Work out the finished part from the listing and answer in its coordinate system (mm). A direction names the side the tool comes from. Round coordinates to 2 decimals unless told otherwise and drop trailing zeros. Loops run counter-clockwise (first coordinate to the right, second up) from the corner with the lowest first, then second, coordinate; pieces in that order, holes last. Notation, with made-up numbers: (51.25, -15) -> (62.25, -15) arc R14 ccw to (62.25, -7) -> close; hole circle Ø8 at (36.5, -12.75). An arc over 180 degrees is marked (long way). Use one line per item in the form item = value.
```python
from build123d import *

# Parameters (mm, degrees)
F0_W     = 14.6
F0_H     = 15
F1_DEPTH = 15
F2_R     = 2
F3_R     = 3
F4_DEPTH = 15.001
F5_SIZE2 = 0.5
F5_SIZE  = 0.5
F9_SIZE2 = 0.5
F9_SIZE  = 0.5


# Not quite as in the source:
# - a pattern or mirror of a feature is missing from the dataset's text; its kind, count and spacing are read off the source's solid


with BuildPart() as f1:
    # F0 (on Right) → F1 (new body)
    with BuildSketch(Plane.YZ):
        Rectangle(F0_W, F0_H)
    extrude(amount=-F1_DEPTH)

    # F2
    f2_edges = [f1.edges().sort_by_distance(p)[0] for p in [
        (-7.5, -7.3, 7.5),
        (-7.5, 7.3, 7.5),
        (-7.5, -7.3, -7.5),
        (-7.5, 7.3, -7.5),
    ]]
    fillet(f2_edges, radius=F2_R)

    # F3 (on face) → F4 (cut, through all)
    with BuildSketch(Plane.YZ):
        Circle(F3_R)
    extrude(amount=-F4_DEPTH, mode=Mode.SUBTRACT)

    # F5
    f5_edges = [f1.edges().sort_by_distance(p)[0] for p in [
        (0, -3, 0),
        (-7.5, 3, 0),
        (-15, -3, 0),
    ]]
    chamfer(f5_edges, length=F5_SIZE, length2=F5_SIZE2)

    # F7 (on mid) → F8 (revolve)
    with BuildSketch(Plane.YZ.offset(-7.5)):
        Polygon((-7.3, 0), (-12.8, 0), (-12.8, -4), (-10.8, -4), (-10.8, -3), (-9.8, -3), (-9.8, -4), (-7.3, -4), align=None)
    f8 = revolve(axis=Axis((-7.5, -3.65, 0), (0, -1, 0)))

    # F8_copies: F8 across plane
    add(f8.mirror(Plane.ZX))

    # F9
    f9_edges = [f1.edges().sort_by_distance(p)[0] for p in [
        (-7.5, -12.8, 4),
        (-7.5, 12.8, 4),
    ]]
    chamfer(f9_edges, length=F9_SIZE, length2=F9_SIZE2)


solid = f1.part
```
(1) Find section C-C, the plane y = -9. Write down the section's boundary in (x, z), then the cut area to 3 significant figures.
Completed:
outline = circle Ø8 at (-7.5, 0)
area = 50.3 mm2
(2) Consider L1, parallel to Z at x = -7.75, y = 0; L2, parallel to Y at x = -9.5, z = 1; L3, parallel to Y at x = -3.75, z = -1.25. Determine where each line is inside the solid, lowest interval first.
Completed:
L1 = -7.5 to -3, 3 to 7.5
L2 = -12.8 to -2.83, 2.83 to 12.8
L3 = -12.35 to -10.8, -9.8 to -2.73, 2.73 to 9.8, 10.8 to 12.35
(3) Find section A-A, the plane y = 0. Write down the section's boundary in (x, z).
Completed:
outline = (-15, -7.5) -> (0, -7.5) -> (0, -3.5) -> (-0.5, -3) -> (-14.5, -3) -> (-15, -3.5) -> close; (-15, 3.5) -> (-14.5, 3) -> (-0.5, 3) -> (0, 3.5) -> (0, 7.5) -> (-15, 7.5) -> close
(4) Given P1, Ø3.5, axis at x = -4, z = -2, coming from the +Y side; P2, Ø1, axis at x = -12, z = 1.5, coming from the +Y side; P3, Ø5.5, axis at y = 0, z = 0, coming from the +X side, each flat-ended and moving along its own axis, determine where each tip first touches the part or whether it passes through.
Completed:
P1 = 12.8
P2 = 7.3
P3 = through
(5) Find section B-B, the plane x = -2.75. Write down the section's boundary in (y, z), then the cut area to 3 significant figures.
Completed:
outline = (-7.3, -5.5) arc R2 ccw to (-5.3, -7.5) -> (5.3, -7.5) arc R2 ccw to (7.3, -5.5) -> (7.3, 5.5) arc R2 ccw to (5.3, 7.5) -> (-5.3, 7.5) arc R2 ccw to (-7.3, 5.5) -> close; hole circle Ø6 at (0, 0)
area = 187 mm2
(6) For a pull along Y with two mould halves and no side action, classify faces 1 (the cylindrical face through (-4.526, -10.293, 0.391)), 2 (the flat face through (0, -3.3, 1.8)), 3 (the cylindrical face through (-7.6, -6.73, 6.9)) as +Y half, -Y half, draft (parallel to the pull), parting line (faces both ways), or undercut.
Completed:
face_1 = undercut
face_2 = draft
face_3 = -Y half
(7) For faces 4 (the cylindrical face through (-6.299, 8.532, -3.815)), 5 (the cylindrical face through (-4.526, 10.293, 0.391)), 6 (the cylindrical face through (-6.299, -8.532, -3.815)), determine the directions among +Z, -Z, +X, -X, +Y, -Y from which every point of the face is accessible in a straight line to the end or side of a thin tool.
Completed:
face_4 = +Y
face_5 = none
face_6 = -Y
